from build123d import *

# Parameters (mm, degrees)
F0_R     = 4.445
F1_DEPTH = 6.35


with BuildPart() as f1:
    # F0 (on Front) → F1 (new body)
    with BuildSketch(Plane.XZ):
        with BuildLine():
            Line((-19.05, 0), (0, 0))
            Line((0, 0), (19.05, 0))
            Line((19.05, 0), (329.55476, 83.1995))
            ThreePointArc((329.55476, 83.1995), (344.977801, 95.034016), (347.515272, 114.308019))
            Line((347.515272, 114.308019), (336.498634, 155.422674))
            ThreePointArc((336.498634, 155.422674), (324.664118, 170.845716), (305.390114, 173.383186))
            Line((305.390114, 173.383186), (27.043501, 98.800436))
            ThreePointArc((27.043501, 98.800436), (21.534365, 99.896271), (19.05, 104.934065))
            Line((19.05, 104.934065), (19.05, 107.662174))
            ThreePointArc((19.05, 107.662174), (20.362206, 111.527809), (23.756499, 113.795803))
            Line((23.756499, 113.795803), (329.55476, 195.7342))
            ThreePointArc((329.55476, 195.7342), (344.977801, 207.568716), (347.515272, 226.842719))
            Line((347.515272, 226.842719), (336.498634, 267.957374))
            ThreePointArc((336.498634, 267.957374), (324.664118, 283.380416), (305.390114, 285.917886))
            Line((305.390114, 285.917886), (27.043501, 211.335136))
            ThreePointArc((27.043501, 211.335136), (21.534365, 212.430971), (19.05, 217.468765))
            Line((19.05, 217.468765), (19.05, 220.196874))
            ThreePointArc((19.05, 220.196874), (20.362206, 224.062509), (23.756499, 226.330503))
            Line((23.756499, 226.330503), (329.55476, 308.2689))
            ThreePointArc((329.55476, 308.2689), (344.977801, 320.103416), (347.515272, 339.377419))
            Line((347.515272, 339.377419), (336.498634, 380.492074))
            ThreePointArc((336.498634, 380.492074), (324.664118, 395.915116), (305.390114, 398.452586))
            Line((305.390114, 398.452586), (27.043501, 323.869836))
            ThreePointArc((27.043501, 323.869836), (21.534365, 324.965671), (19.05, 330.003465))
            Line((19.05, 330.003465), (19.05, 332.731574))
            ThreePointArc((19.05, 332.731574), (20.362206, 336.597209), (23.756499, 338.865203))
            Line((23.756499, 338.865203), (329.55476, 420.8036))
            ThreePointArc((329.55476, 420.8036), (344.977801, 432.638116), (347.515272, 451.912119))
            Line((347.515272, 451.912119), (336.498634, 493.026774))
            ThreePointArc((336.498634, 493.026774), (324.664118, 508.449816), (305.390114, 510.987286))
            Line((305.390114, 510.987286), (27.043501, 436.404536))
            ThreePointArc((27.043501, 436.404536), (21.534365, 437.500371), (19.05, 442.538165))
            Line((19.05, 442.538165), (19.05, 445.266274))
            ThreePointArc((19.05, 445.266274), (20.362206, 449.131909), (23.756499, 451.399903))
            Line((23.756499, 451.399903), (329.55476, 533.3383))
            ThreePointArc((329.55476, 533.3383), (344.977801, 545.172816), (347.515272, 564.446819))
            Line((347.515272, 564.446819), (336.498634, 605.561474))
            ThreePointArc((336.498634, 605.561474), (324.664118, 620.984516), (305.390114, 623.521986))
            Line((305.390114, 623.521986), (27.043501, 548.939236))
            ThreePointArc((27.043501, 548.939236), (21.534365, 550.035071), (19.05, 555.072865))
            Line((19.05, 555.072865), (19.05, 557.800974))
            ThreePointArc((19.05, 557.800974), (20.362206, 561.666609), (23.756499, 563.934603))
            Line((23.756499, 563.934603), (329.55476, 645.873))
            ThreePointArc((329.55476, 645.873), (344.977801, 657.707516), (347.515272, 676.981519))
            Line((347.515272, 676.981519), (336.498634, 718.096174))
            ThreePointArc((336.498634, 718.096174), (324.664118, 733.519216), (305.390114, 736.056686))
            Line((305.390114, 736.056686), (27.043501, 661.473936))
            ThreePointArc((27.043501, 661.473936), (21.534365, 662.569771), (19.05, 667.607565))
            Line((19.05, 667.607565), (19.05, 670.335674))
            ThreePointArc((19.05, 670.335674), (20.362206, 674.201309), (23.756499, 676.469303))
            Line((23.756499, 676.469303), (329.55476, 758.4077))
            ThreePointArc((329.55476, 758.4077), (344.977801, 770.242216), (347.515272, 789.516219))
            Line((347.515272, 789.516219), (336.498634, 830.630874))
            ThreePointArc((336.498634, 830.630874), (324.664118, 846.053916), (305.390114, 848.591386))
            Line((305.390114, 848.591386), (27.043501, 774.008636))
            ThreePointArc((27.043501, 774.008636), (21.534365, 775.104471), (19.05, 780.142265))
            Line((19.05, 780.142265), (19.05, 782.870374))
            ThreePointArc((19.05, 782.870374), (20.362206, 786.736009), (23.756499, 789.004003))
            Line((23.756499, 789.004003), (329.55476, 870.9424))
            ThreePointArc((329.55476, 870.9424), (344.977801, 882.776916), (347.515272, 902.050919))
            Line((347.515272, 902.050919), (336.498634, 943.165574))
            ThreePointArc((336.498634, 943.165574), (324.664118, 958.588616), (305.390114, 961.126086))
            Line((305.390114, 961.126086), (0, 879.297052))
            Line((0, 879.297052), (-305.390114, 961.126086))
            ThreePointArc((-305.390114, 961.126086), (-324.664118, 958.588616), (-336.498634, 943.165574))
            Line((-336.498634, 943.165574), (-347.515272, 902.050919))
            ThreePointArc((-347.515272, 902.050919), (-344.977801, 882.776916), (-329.55476, 870.9424))
            Line((-329.55476, 870.9424), (-23.756499, 789.004003))
            ThreePointArc((-23.756499, 789.004003), (-20.362206, 786.736009), (-19.05, 782.870374))
            Line((-19.05, 782.870374), (-19.05, 780.142265))
            ThreePointArc((-19.05, 780.142265), (-21.534365, 775.104471), (-27.043501, 774.008636))
            Line((-27.043501, 774.008636), (-305.390114, 848.591386))
            ThreePointArc((-305.390114, 848.591386), (-324.664118, 846.053916), (-336.498634, 830.630874))
            Line((-336.498634, 830.630874), (-347.515272, 789.516219))
            ThreePointArc((-347.515272, 789.516219), (-344.977801, 770.242216), (-329.55476, 758.4077))
            Line((-329.55476, 758.4077), (-23.756499, 676.469303))
            ThreePointArc((-23.756499, 676.469303), (-20.362206, 674.201309), (-19.05, 670.335674))
            Line((-19.05, 670.335674), (-19.05, 667.607565))
            ThreePointArc((-19.05, 667.607565), (-21.534365, 662.569771), (-27.043501, 661.473936))
            Line((-27.043501, 661.473936), (-305.390114, 736.056686))
            ThreePointArc((-305.390114, 736.056686), (-324.664118, 733.519216), (-336.498634, 718.096174))
            Line((-336.498634, 718.096174), (-347.515272, 676.981519))
            ThreePointArc((-347.515272, 676.981519), (-344.977801, 657.707516), (-329.55476, 645.873))
            Line((-329.55476, 645.873), (-23.756499, 563.934603))
            ThreePointArc((-23.756499, 563.934603), (-20.362206, 561.666609), (-19.05, 557.800974))
            Line((-19.05, 557.800974), (-19.05, 555.072865))
            ThreePointArc((-19.05, 555.072865), (-21.534365, 550.035071), (-27.043501, 548.939236))
            Line((-27.043501, 548.939236), (-305.390114, 623.521986))
            ThreePointArc((-305.390114, 623.521986), (-324.664118, 620.984516), (-336.498634, 605.561474))
            Line((-336.498634, 605.561474), (-347.515272, 564.446819))
            ThreePointArc((-347.515272, 564.446819), (-344.977801, 545.172816), (-329.55476, 533.3383))
            Line((-329.55476, 533.3383), (-23.756499, 451.399903))
            ThreePointArc((-23.756499, 451.399903), (-20.362206, 449.131909), (-19.05, 445.266274))
            Line((-19.05, 445.266274), (-19.05, 442.538165))
            ThreePointArc((-19.05, 442.538165), (-21.534365, 437.500371), (-27.043501, 436.404536))
            Line((-27.043501, 436.404536), (-305.390114, 510.987286))
            ThreePointArc((-305.390114, 510.987286), (-324.664118, 508.449816), (-336.498634, 493.026774))
            Line((-336.498634, 493.026774), (-347.515272, 451.912119))
            ThreePointArc((-347.515272, 451.912119), (-344.977801, 432.638116), (-329.55476, 420.8036))
            Line((-329.55476, 420.8036), (-23.756499, 338.865203))
            ThreePointArc((-23.756499, 338.865203), (-20.362206, 336.597209), (-19.05, 332.731574))
            Line((-19.05, 332.731574), (-19.05, 330.003465))
            ThreePointArc((-19.05, 330.003465), (-21.534365, 324.965671), (-27.043501, 323.869836))
            Line((-27.043501, 323.869836), (-305.390114, 398.452586))
            ThreePointArc((-305.390114, 398.452586), (-324.664118, 395.915116), (-336.498634, 380.492074))
            Line((-336.498634, 380.492074), (-347.515272, 339.377419))
            ThreePointArc((-347.515272, 339.377419), (-344.977801, 320.103416), (-329.55476, 308.2689))
            Line((-329.55476, 308.2689), (-23.756499, 226.330503))
            ThreePointArc((-23.756499, 226.330503), (-20.362206, 224.062509), (-19.05, 220.196874))
            Line((-19.05, 220.196874), (-19.05, 217.468765))
            ThreePointArc((-19.05, 217.468765), (-21.534365, 212.430971), (-27.043501, 211.335136))
            Line((-27.043501, 211.335136), (-305.390114, 285.917886))
            ThreePointArc((-305.390114, 285.917886), (-324.664118, 283.380416), (-336.498634, 267.957374))
            Line((-336.498634, 267.957374), (-347.515272, 226.842719))
            ThreePointArc((-347.515272, 226.842719), (-344.977801, 207.568716), (-329.55476, 195.7342))
            Line((-329.55476, 195.7342), (-23.756499, 113.795803))
            ThreePointArc((-23.756499, 113.795803), (-20.362206, 111.527809), (-19.05, 107.662174))
            Line((-19.05, 107.662174), (-19.05, 104.934065))
            ThreePointArc((-19.05, 104.934065), (-21.534365, 99.896271), (-27.043501, 98.800436))
            Line((-27.043501, 98.800436), (-305.390114, 173.383186))
            ThreePointArc((-305.390114, 173.383186), (-324.664118, 170.845716), (-336.498634, 155.422674))
            Line((-336.498634, 155.422674), (-347.515272, 114.308019))
            ThreePointArc((-347.515272, 114.308019), (-344.977801, 95.034016), (-329.55476, 83.1995))
            Line((-329.55476, 83.1995), (-19.05, 0))
        make_face()
        with Locations((0, 50.8)):
            Circle(F0_R, mode=Mode.SUBTRACT)
        with Locations((0, 828.497052)):
            Circle(F0_R, mode=Mode.SUBTRACT)
    extrude(amount=F1_DEPTH)


solid = f1.part
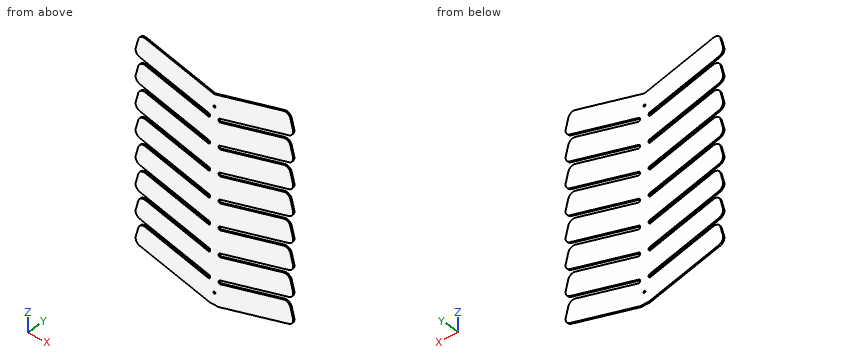
Verification items for the finished model (mm, model axes). Give positions to 0.01 mm unless a question says otherwise; leave off trailing zeros. Order: outer loops, then holes, each group sorted by start corner. A loop starts at its lowest first (then second) coordinate and runs counter-clockwise, first axis right, second up. Notation, with made-up numbers: M -30,78.25 L 28,78.25 A19 cw 28,103.25 Z; hole C -19.5,44 d11. An arc over 180 degrees is marked long. Answer as a JSON object with one key per item and string values. Group by question number.
1) Cross-section at C-C (z = 365). Enter the section's corners in (x, y), then the cut area to 3 significant figures.
2) Scan lines: line 1 along Z through (x, y) = (0, -3.5) (3 decimals); line 2 along Z through (x, y) = (-4, -4.25). Record each from-to range of solid material in increasing order. Write a range as [from, to].
3) Depth check by flat-ended pin: pin 1 Ø3 at (y, z) = (-1, 696) entering from -X; pin 2 Ø2 at (y, z) = (-4, 668.5) entering from -X; pin 3 Ø0.8 at (y, z) = (-4, 781.5) entering from +X; pin 4 Ø3 at (x, z) = (76.5, 866) entering from +Y. Enter the tip coordinate at first touch or a pass-through.
4) Cross-section at B-B (x = -272.5). Give the number of separate pieces and of enclosed holes in the cut face, then the cut area to 3 significant figures.
5) Cross-section at A-A (z = 889). Enter the section's corners in (x, y).
Result sheet:
{
 "1": {"outline": "M -340.65,-6.35 L -180.54,-6.35 L -180.54,0 L -340.65,0 Z; M -121.29,-6.35 L 121.29,-6.35 L 121.29,0 L -121.29,0 Z; M 180.54,-6.35 L 340.65,-6.35 L 340.65,0 L 180.54,0 Z", "area": "3,570 mm2"},
 "2": {"line 1": "z = [0, 46.355], [55.245, 824.052], [832.942, 879.297]", "line 2": "z = [0, 48.86], [52.74, 826.56], [830.44, 880.37]"},
 "3": {"pin 1": "stops at x = -342.82", "pin 2": "stops at x = -348.36", "pin 3": "stops at x = 348.36", "pin 4": "stops at y = 0"},
 "4": {"separate pieces": "8", "enclosed holes": "0", "area": "4,910 mm2"},
 "5": {"outline": "M -347.54,-6.35 L -36.21,-6.35 L -36.21,0 L -347.54,0 Z; M 36.21,-6.35 L 347.54,-6.35 L 347.54,0 L 36.21,0 Z"}
}
